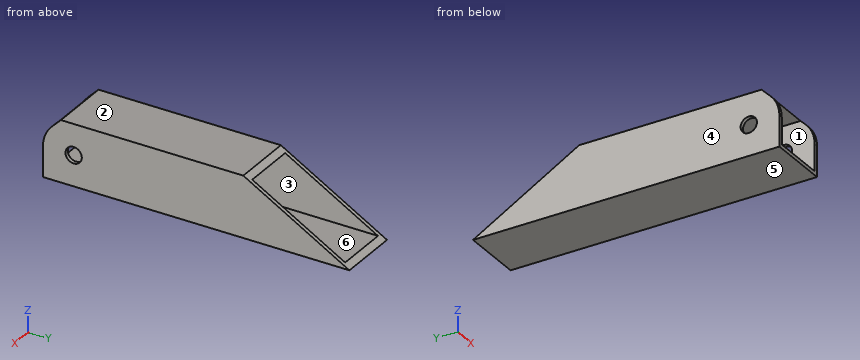
```python
from build123d import *

# Parameters (mm, degrees)
SKETCH1_W               = 25.4
SKETCH1_H               = 25.4
SKETCH1_W_2             = 22.225
SKETCH1_H_2             = 22.225
EXTRUDE1_DEPTH          = 127
EXTRUDE3_DEPTH          = 131.136274728
F_1_4_CLEARANCE_HOLE1_D = 6.7564
EXTRUDE4_DEPTH          = 131.136274728
EXTRUDE5_DEPTH          = 131.136274728


with BuildPart() as part:
    # Sketch1 → Extrude1 (new body)
    with BuildSketch(Plane(origin=(0, 0, 0), x_dir=(1, 0, 0), z_dir=(0, 1, 0))):
        Rectangle(SKETCH1_W, SKETCH1_H)
        Rectangle(SKETCH1_W_2, SKETCH1_H_2, mode=Mode.SUBTRACT)
    extrude(amount=EXTRUDE1_DEPTH)

    # Sketch3 → Extrude3 (cut, through all)
    with BuildSketch(Plane(origin=(12.7, 0, 0), x_dir=(0, 0, -1), z_dir=(1, 0, 0))):
        Polygon((12.7, 127), (-12.7, 127), (-12.7, 83.005909488), align=None)
    extrude(amount=-EXTRUDE3_DEPTH, mode=Mode.SUBTRACT)

    # 1/4 Clearance Hole1 (through all)
    with Locations(Plane(origin=(12.7, 0, 0), x_dir=(0, 0, -1), z_dir=(1, 0, 0))):
        with Locations((0, 12.7)):
            Hole(F_1_4_CLEARANCE_HOLE1_D / 2)

    # Sketch7 → Extrude4 (cut, through all)
    with BuildSketch(Plane(origin=(12.7, 0, 0), x_dir=(0, 0, -1), z_dir=(1, 0, 0))):
        Polygon((-5.260512242, 0), (-12.7, 7.439487758), (-12.7, 0), align=None)
    extrude(amount=-EXTRUDE4_DEPTH, mode=Mode.SUBTRACT)

    # Sketch8 → Extrude5 (cut, through all)
    with BuildSketch(Plane(origin=(12.7, 0, 0), x_dir=(0, 0, -1), z_dir=(1, 0, 0))):
        with BuildLine():
            Line((0, 0), (-5.260512242, 0))
            Line((-5.260512242, 0), (-8.980256121, 3.719743879))
            ThreePointArc((-8.980256121, 3.719743879), (-4.860079591, 0.966729937), (0, 0))
        make_face()
    extrude(amount=-EXTRUDE5_DEPTH, mode=Mode.SUBTRACT)


solid = part.part
```
Model file for the job. Use its own axes, mm. Face numbers are marked on the shaded views. A direction names the side the tool comes from. Give positions to 0.01 mm unless a question says otherwise; leave off trailing zeros. Write each loop counter-clockwise with the first axis right and the second up, starting at its lowest first coordinate (ties: lowest second). Pieces come first, ordered by that corner, then holes. Notation, with made-up numbers: (47.5, -27.75) - (70.5, -27.75) arc R25 ccw to (70.5, 9.25) - close; hole circle Ø9 at (36, 26.25). An arc over 180 degrees is marked (long way). One line per question, with ' | ' between items. Start each with the question number.
(1) Slice it at C-C on y = 12.7. Write the cut outline in (x, z), plus the area to 3 significant figures.
(2) Pin check, flat tips, straight feed: P1, Ø1, axis at x = -3.5, y = 110, coming from the +Z side; P2, Ø9, axis at y = 12.7, z = 0, coming from the -X side. Stop position of each tip, or through.
(3) Slice it at A-A on x = -6.75. Write the cut outline in (y, z).
(4) Wall check: line 1 along Z through (x, y) = (9.5, 40.5); line 2 along Z through (x, y) = (0.5, 117). Give the ranges that are in metal, low to high. Write a range as from..to.
(5) 3-axis set-ups, long thin cutter, end or side, ignore diameter. For the marked faces 5 and 6: which of +Z, -Z, +X, -X, +Y, -Y reach the whole face in a straight line?
(6) Slice it at B-B on y = 46. Write the cut outline in (x, z).
(7) Slice it at D-D on z = -8.5. Write the cut outline in (x, y), plus the area to 3 significant figures.
(8) Two-plate mould, pull along X, no slides. Class the marked faces 1, 2, 3 and 4: +X half, -X half, draft (parallel to the pull), parting line (faces both ways), or undercut.
Results below:
1) outline: (-12.7, -12.7) - (12.7, -12.7) - (12.7, -3.38) - (11.11, -3.38) - (11.11, -11.11) - (-11.11, -11.11) - (-11.11, -3.38) - (-12.7, -3.38) - close; (-12.7, 3.38) - (-11.11, 3.38) - (-11.11, 11.11) - (11.11, 11.11) - (11.11, 3.38) - (12.7, 3.38) - (12.7, 12.7) - (-12.7, 12.7) - close | area: 130 mm^2
2) P1: z = -11.11 | P2: x = -12.7
3) outline: (0, -12.7) - (127, -12.7) - (124.25, -11.11) - (0, -11.11) - close; (5.85, 11.11) - (85.76, 11.11) - (83.01, 12.7) - (7.44, 12.7) - close
4) line 1: -12.7..-11.11, 11.11..12.7 | line 2: -12.7..-11.11
5) face 5: -Z, +X, -X, +Y, -Y | face 6: +Y, -Y
6) outline: (-12.7, -12.7) - (12.7, -12.7) - (12.7, 12.7) - (-12.7, 12.7) - close; hole (-11.11, -11.11) - (11.11, -11.11) - (11.11, 11.11) - (-11.11, 11.11) - close
7) outline: (-12.7, 0) - (-11.11, 0) - (-11.11, 119.73) - (-12.7, 119.73) - close; (11.11, 0) - (12.7, 0) - (12.7, 119.73) - (11.11, 119.73) - close | area: 380 mm^2
8) face 1: undercut | face 2: draft | face 3: undercut | face 4: -X half
